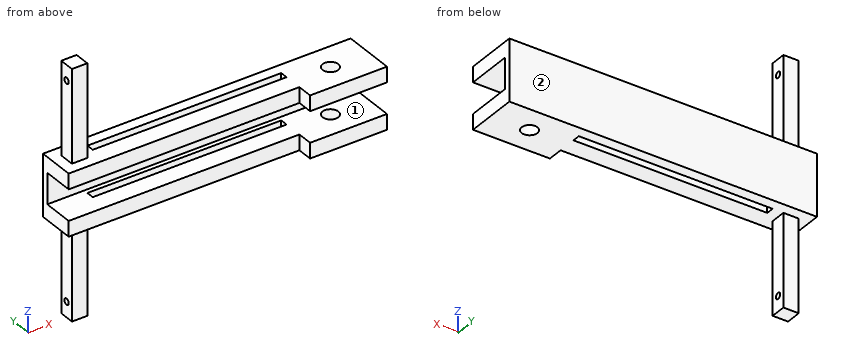
from build123d import *

# Parameters (mm, degrees)
F0_W      = 254
F0_H      = 50.8
F1_DEPTH  = 30.48
F2_W      = 254
F2_H      = 25.4
F3_DEPTH  = 25.4
F4_W      = 12.7
F4_H      = 12.7
F6_DEPTH  = 76.2
F5_W      = 12.7
F5_H      = 12.7
F7_DEPTH  = 76.2
F8_W      = 63.5
F8_H      = 12.7
F10_DEPTH = 12.7
F9_W      = 63.5
F9_H      = 12.7
F11_DEPTH = 12.7
F12_W     = 160.02
F12_H     = 6.35
F14_DEPTH = 127.001
F13_R     = 6.477
F15_DEPTH = 127.001
F16_R     = 2.54
F18_DEPTH = 25.4
F17_R     = 2.54
F19_DEPTH = 25.4


with BuildPart() as f1:
    # F0 (on Front) → F1 (new body)
    with BuildSketch(Plane.XZ):
        with Locations((-4.6371974824, 18.0667741224)):
            Rectangle(F0_W, F0_H)
    extrude(amount=F1_DEPTH)

    # F2 (on face) → F3 (cut)
    with BuildSketch(Plane.XZ.offset(30.48)):
        with Locations((-4.6371974824, 18.0667741224)):
            Rectangle(F2_W, F2_H)
    extrude(amount=-F3_DEPTH, mode=Mode.SUBTRACT)

    # F4 (on face) → F6 (join)
    with BuildSketch(Plane(origin=(0, 0, -7.3332258776), x_dir=(1, 0, 0), z_dir=(0, 0, -1))):
        with Locations((-116.3971974824, 15.24)):
            Rectangle(F4_W, F4_H)
    extrude(amount=F6_DEPTH)

    # F5 (on face) → F7 (join)
    with BuildSketch(Plane.XY.offset(43.4667741224)):
        with Locations((-116.3971974824, -15.24)):
            Rectangle(F5_W, F5_H)
    extrude(amount=F7_DEPTH)

    # F8 (on face) → F10 (join)
    with BuildSketch(Plane.XZ.offset(30.48)):
        with Locations((90.6128025176, 37.1167741224)):
            Rectangle(F8_W, F8_H)
    extrude(amount=F10_DEPTH)

    # F9 (on face) → F11 (join)
    with BuildSketch(Plane.XZ.offset(30.48)):
        with Locations((90.6128025176, -0.9832258776)):
            Rectangle(F9_W, F9_H)
    extrude(amount=F11_DEPTH)

    # F12 (on face) → F14 (cut, through all)
    with BuildSketch(Plane(origin=(0, 0, -7.3332258776), x_dir=(1, 0, 0), z_dir=(0, 0, -1))):
        with Locations((-21.1471974824, 12.065)):
            Rectangle(F12_W, F12_H)
    extrude(amount=-F14_DEPTH, mode=Mode.SUBTRACT)

    # F13 (on face) → F15 (cut, through all)
    with BuildSketch(Plane(origin=(0, 0, -7.3332258776), x_dir=(1, 0, 0), z_dir=(0, 0, -1))):
        with Locations((90.6128025176, 21.7048414052)):
            Circle(F13_R)
    extrude(amount=-F15_DEPTH, mode=Mode.SUBTRACT)

    # F16 (on face) → F18 (cut)
    with BuildSketch(Plane.YZ.offset(-110.0471974824)):
        with Locations((-15.24, -70.8332258776)):
            Circle(F16_R)
    extrude(amount=-F18_DEPTH, mode=Mode.SUBTRACT)

    # F17 (on face) → F19 (cut)
    with BuildSketch(Plane.YZ.offset(-110.0471974824)):
        with Locations((-15.24, 106.9667741224)):
            Circle(F17_R)
    extrude(amount=-F19_DEPTH, mode=Mode.SUBTRACT)


solid = f1.part
Here's how the part is built. I have some questions about the finished solid (model axes, mm). Face numbers are marked on the shaded views. A direction names the side the tool comes from. Round coordinates to 2 decimals unless told otherwise and drop trailing zeros. Loops run counter-clockwise (first coordinate to the right, second up) from the corner with the lowest first, then second, coordinate; pieces in that order, holes last. Notation, with made-up numbers: M 72,7.5 L 124,7.5 A22 ccw 124,46.5 Z; hole C 38,-33.5 d7. An arc over 180 degrees is marked long. Write each question's results on one line, items separated by ' | '. Start each with the question number.
(1) On a 3-axis mill with a long thin cutter (end or side, diameter ignored), from which of +Z, -Z, +X, -X, +Y, -Y can I reach the whole of each face in a straight line? I mean the marked faces 1 and 2. Say none if no direction works.
(2) I want a section at D-D (x = 67). Please give me the cut outline in (y, z), then the cut area to 3 significant figures.
(3) I want a section at C-C (z = 34). Please give me the cut outline in (x, y), then the cut area to 3 significant figures.
(4) If I drill on probe 1 along Z at (x, y) = (-109, -24); probe 2 along Y at (x, z) = (-7.5, 5); probe 3 along X at (y, z) = (-19.5, -56.5), over which ranges is the centre line in solid material (lowest first)? Write a range as from..to.
(5) I want a section at A-A (x = 41). Please give me the cut outline in (y, z).
(6) I want a section at B-B (y = -35). Please give me the cut outline in (x, z), then the cut area to 3 significant figures.
(7) Will these pins go through, and if not, where does the flat tip stop? P1, Ø6.5, axis at y = -14, z = -34.5, coming from the -X side; P2, Ø5, axis at y = -22.5, z = -37.5, coming from the +X side; P3, Ø8, axis at x = 23.5, y = -27, coming from the -Z side; P4, Ø11.5, axis at x = 90.61, y = -21.7, coming from the +Z side.
Solved:
1) face 1: +X, -X, -Y | face 2: +Z, -Z, +X, -X, +Y
2) outline: M -43.18,-7.33 L 0,-7.33 L 0,43.47 L -43.18,43.47 L -43.18,30.77 L -5.08,30.77 L -5.08,5.37 L -43.18,5.37 Z | area: 1,230 mm²
3) outline: M -131.64,-30.48 L 58.86,-30.48 L 58.86,-43.18 L 122.36,-43.18 L 122.36,0 L -131.64,0 Z; hole M -101.16,-15.24 L 58.86,-15.24 L 58.86,-8.89 L -101.16,-8.89 Z; hole C 90.61,-21.7 d12.95 | area: 7,400 mm²
4) probe 1: z = -7.33..5.37, 30.77..43.47 | probe 2: y = -30.48..-15.24, -8.89..0 | probe 3: x = -122.75..-110.05
5) outline: M -30.48,-7.33 L -15.24,-7.33 L -15.24,5.37 L -30.48,5.37 Z; M -30.48,30.77 L -15.24,30.77 L -15.24,43.47 L -30.48,43.47 Z; M -8.89,-7.33 L 0,-7.33 L 0,43.47 L -8.89,43.47 L -8.89,30.77 L -5.08,30.77 L -5.08,5.37 L -8.89,5.37 Z
6) outline: M 58.86,-7.33 L 122.36,-7.33 L 122.36,5.37 L 58.86,5.37 Z; M 58.86,30.77 L 122.36,30.77 L 122.36,43.47 L 58.86,43.47 Z | area: 1,610 mm²
7) P1: stops at x = -122.75 | P2: stops at x = -110.05 | P3: stops at z = -7.33 | P4: passes through
